```python
from build123d import *

# Parameters (mm, degrees)
BOSS_EXTRUDE1_DEPTH     = 5
CHAMFER1_SIZE           = 2
BOSS_EXTRUDE4_START     = 80
BOSS_EXTRUDE4_OUTLINE_W = 26
BOSS_EXTRUDE4_OUTLINE_H = 5
BOSS_EXTRUDE4_DEPTH     = 3
SKETCH2_R               = 4.1
SKETCH2_R_2             = 4
CUT_EXTRUDE2_DEPTH      = 36.925038653
SKETCH4_R               = 4.1
CUT_EXTRUDE3_DEPTH      = 9.191294825
SKETCH5_W               = 174
SKETCH5_H               = 5
BOSS_EXTRUDE5_DEPTH     = 50


with BuildPart() as part:
    # Boss-Extrude1: read off the stored shape, not the designer's step
    # Boss-Extrude1 outline → Boss-Extrude1 (new body)
    with BuildSketch(Plane.XY):
        Polygon((-87, 62), (-80.501435369, -62), (80.501435369, -62), (87, 62), (87, 86), (73.257786703, 86), (73.257786703, 83), (47.257786703, 83), (47.257786703, 90), (87, 90), (87, 112), (-87, 112), (-87, 90), (-47.257786703, 90), (-47.257786703, 83), (-73.257786703, 83), (-73.257786703, 86), (-87, 86), align=None)
        with BuildLine():
            Line((-25, -17), (25, -17))
            ThreePointArc((25, -17), (45, -37), (25, -57))
            Line((25, -57), (-25, -57))
            ThreePointArc((-25, -57), (-45, -37), (-25, -17))
        make_face(mode=Mode.SUBTRACT)
    extrude(amount=BOSS_EXTRUDE1_DEPTH)

    # Chamfer1
    chamfer1_edges = [part.edges().sort_by_distance(p)[0] for p in [
        (60.257786703, 83, 5),
        (-60.257786703, 83, 5),
    ]]
    chamfer(chamfer1_edges, length=CHAMFER1_SIZE)

    # Boss-Extrude4: read off the stored shape, not the designer's step
    # Boss-Extrude4 outline → Boss-Extrude4 (add)
    with BuildSketch(Plane(origin=(0, 0, 0), x_dir=(1, 0, 0), z_dir=(0, 1, 0)).offset(BOSS_EXTRUDE4_START)):
        with Locations((60.257786703, -2.5)):
            Rectangle(BOSS_EXTRUDE4_OUTLINE_W, BOSS_EXTRUDE4_OUTLINE_H)
        with Locations((-60.257786703, -2.5)):
            Rectangle(BOSS_EXTRUDE4_OUTLINE_W, BOSS_EXTRUDE4_OUTLINE_H)
    extrude(amount=BOSS_EXTRUDE4_DEPTH)

    # Sketch2 → Cut-Extrude2 (cut)
    with BuildSketch(Plane.XY.offset(5)):
        with Locations((-62.28149578, 27.917996168)):
            Circle(SKETCH2_R)
        with Locations((62.28149578, 27.917996168)):
            Circle(SKETCH2_R_2)
    extrude(amount=-CUT_EXTRUDE2_DEPTH, mode=Mode.SUBTRACT)

    # Sketch4 → Cut-Extrude3 (cut)
    with BuildSketch(Plane(origin=(0, 0, 0), x_dir=(-1, 0, 0), z_dir=(0, 0, -1))):
        with Locations((-47.001300636, -11.749189401)):
            Circle(SKETCH4_R)
        with Locations((47.999909157, -11.750133675)):
            Circle(SKETCH4_R)
        with Locations((47.999996185, -54.249608673)):
            Circle(SKETCH4_R)
        with Locations((-46.999683563, -54.249320844)):
            Circle(SKETCH4_R)
    extrude(amount=-CUT_EXTRUDE3_DEPTH, mode=Mode.SUBTRACT)

    # Sketch5 → Boss-Extrude5 (add)
    with BuildSketch(Plane(origin=(0, 112, 0), x_dir=(1, 0, 0), z_dir=(0, 1, 0))):
        with Locations((0, -2.5)):
            Rectangle(SKETCH5_W, SKETCH5_H)
    extrude(amount=BOSS_EXTRUDE5_DEPTH)


solid = part.part
```
For this review, take the finished solid that the model builds, in its own axes (mm). A direction names the side the tool comes from. Round coordinates to 2 decimals unless told otherwise and drop trailing zeros. Write each loop counter-clockwise with the first axis right and the second up, starting at its lowest first coordinate (ties: lowest second). Pieces come first, ordered by that corner, then holes. Notation, with made-up numbers: M 50.5,23 L 100.5,23 A18 cw 100.5,39 Z; hole C 66.25,27 d11. An arc over 180 degrees is marked long. One line per item, written item: value. Start each with the question number.
(1) Wall thickness on line 1 (Y direction, x = 74, z = 3.65); line 2 (Y direction, x = 1, z = 1.5); line 3 (X direction, y = 31.5, z = 1.3): over which ranges is each line inside the solid? List them lowest first.
(2) We need section B-B (y = -37). Give the boundary of the cut face in (x, z).
(3) We need section A-A (x = -5). Give the boundary of the cut face in (y, z), and give its area (3 significant figures).
(4) We need section C-C (x = 62). Give the boundary of the cut face in (y, z).
(5) The part is to be moulded in two halves that separate along Y. For faces 4 (the flat face through (-87, 74, 2)), 5 (the flat face through (-1, -62, 2)), 6 (the flat face through (80, 86, 2)), say which applies: released by +Y, released by -Y, zero draft, split by the parting line, or undercut.
(6) Machinability: for faces 1 (the flat face through (-67, 90, 2)), 2 (the flat face through (0, -57, 2)), 3 (the flat face through (-1, 48, 0)), which of the approach directions +Z, -Z, +X, -X, +Y, -Y give a long, thin tool a straight path to every point of the face, cutting with its end or side? Answer none if there is none.
(7) We need section D-D (z = 0.85). Give the boundary of the cut face in (x, y).
Result:
1. line 1: -62 to 86, 90 to 162
1. line 2: -62 to -57, -17 to 162
1. line 3: -85.4 to -64.28, -60.29 to 60.5, 64.06 to 85.4
2. outline: M -81.81,0 L -45,0 L -45,5 L -81.81,5 Z; M 45,0 L 81.81,0 L 81.81,5 L 45,5 Z
3. outline: M -62,0 L -57,0 L -57,5 L -62,5 Z; M -17,0 L 162,0 L 162,5 L -17,5 Z
3. area: 920 mm²
4. outline: M -62,0 L 23.93,0 L 23.93,5 L -62,5 Z; M 31.91,0 L 83,0 L 83,5 L 31.91,5 Z; M 90,0 L 162,0 L 162,5 L 90,5 Z
5. face 4: zero draft
5. face 5: released by -Y
5. face 6: undercut
6. face 1: +Z, -Z, -X
6. face 2: +Z, -Z
6. face 3: -Z, +X, -X, +Y, -Y
7. outline: M -87,62 L -80.5,-62 L 80.5,-62 L 87,62 L 87,86 L 73.26,86 L 73.26,83 L 47.26,83 L 47.26,90 L 87,90 L 87,162 L -87,162 L -87,90 L -47.26,90 L -47.26,83 L -73.26,83 L -73.26,86 L -87,86 Z; hole C -62.28,27.92 d8.2; hole C -48,-54.25 d8.2; hole C -48,-11.75 d8.2; hole M -25,-57 L 25,-57 A20 ccw 25,-17 L -25,-17 A20 ccw Z; hole C 47,-54.25 d8.2; hole C 47,-11.75 d8.2; hole C 62.28,27.92 d8
